The figure shows three views and two pictorial views of one solid part (mm, origin at its lowest corner). Answer the questions. A direction names the side the tool comes from. Give positions to 0.01 mm unless a question says otherwise; leave off trailing zeros. Loops run counter-clockwise (first coordinate to the right, second up) from the corner with the lowest first, then second, coordinate; pieces in that order, holes last. Notation, with made-up numbers: M -23,44 L -19,44 A9 cw -19,59 Z; hole C 36.25,88.25 d3. An arc over 180 degrees is marked long. One line per item, written item: value. Start each with the question number.
Q1. The mould has two halves that part along Z. Classify the marked faces 1, 2 and 3: +Z half, -Z half, draft (parallel to the pull), parting line (faces both ways), or undercut.
Q2. For the marked faces 4, 5, 6 and 7, determine the directions among +Z, -Z, +X, -X, +Y, -Y from which every point of the face is accessible in a straight line to the end or side of a thin tool.
Q3. A cutting plane is placed at A-A, the plane y = 1.4. State how many separate pieces and enclosed holes the cut face has, and give its area (3 significant figures).
Q4. Consider L1, parallel to Y at x = 1.4, z = 2.5; L2, parallel to Y at x = 2.6, z = 2.75 (1 decimal); L3, parallel to X at y = 2.3, z = 10. Determine where each line is inside the solid, lowest interval first.
Q5. A cutting plane is placed at C-C, the plane z = 1.75. Determine the outline of the cut face in (x, y).
Q6. A flat-ended cylindrical pin translates along its axis: pin 1 (1.4 mm diameter, centred on y = 2.5, z = 9.5, fed in from -X). Find the tip coordinate at first contact, or state that the pin passes through.
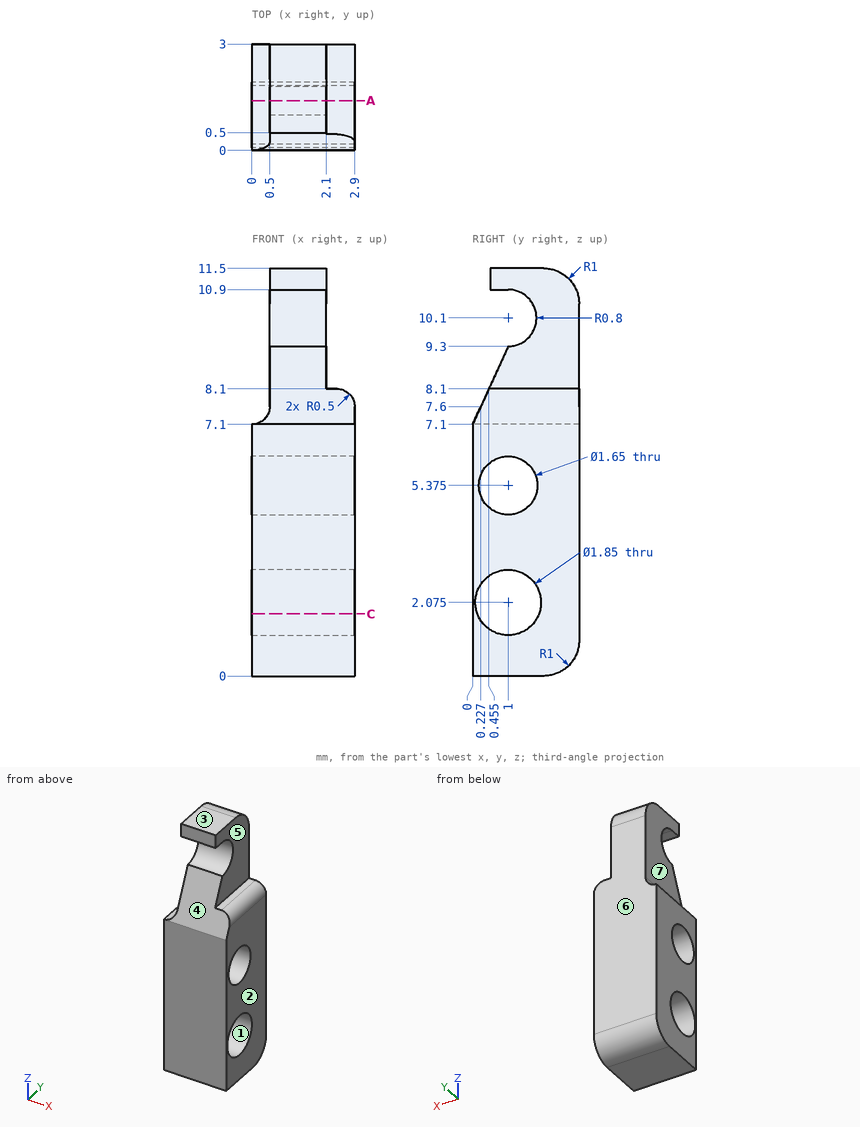
Answer block:
1. face 1: undercut
1. face 2: draft
1. face 3: +Z half
2. face 4: +X, -X, -Y
2. face 5: +Z, +X, +Y, -Y
2. face 6: +Z, -Z, +X, -X, +Y
2. face 7: +Z, -X, +Y, -Y
3. separate pieces: 4
3. enclosed holes: 0
3. area: 17.2 mm^2
4. L1: 0 to 0.18, 1.82 to 3
4. L2: 0 to 0.4, 1.6 to 3
4. L3: 0.5 to 2.1
5. outline: M 0,0 L 2.9,0 L 2.9,0.13 L 0,0.13 Z; M 0,1.87 L 2.9,1.87 L 2.9,3 L 0,3 Z
6. pin 1: x = 0.5
